CAD build for the part. Positions are in the model's coordinates, mm. Round coordinates to 2 decimals unless told otherwise and drop trailing zeros. Loops run counter-clockwise (first coordinate to the right, second up) from the corner with the lowest first, then second, coordinate; pieces in that order, holes last.
from build123d import *

# Parameters (mm, degrees)
SKETCH_W      = 56
SKETCH_H      = 306
PAD_DEPTH     = 3
SKETCH001_W   = 8
SKETCH001_H   = 3
SKETCH001_W_2 = 3
SKETCH001_H_2 = 20
POCKET_DEPTH  = 3.001


with BuildPart() as part:
    # Sketch → Pad (new body)
    with BuildSketch(Plane.XY):
        with Locations((28, 153)):
            Rectangle(SKETCH_W, SKETCH_H)
    extrude(amount=PAD_DEPTH)

    # Sketch001 (on Face6 of Pad) → Pocket (cut, through all)
    with BuildSketch(Plane.XY.offset(3)):
        with Locations((4, 1.5)):
            Rectangle(SKETCH001_W, SKETCH001_H)
        with Locations((20, 1.5)):
            Rectangle(SKETCH001_W, SKETCH001_H)
        with Locations((36, 1.5)):
            Rectangle(SKETCH001_W, SKETCH001_H)
        with Locations((52, 1.5)):
            Rectangle(SKETCH001_W, SKETCH001_H)
        with Locations((4, 304.5)):
            Rectangle(SKETCH001_W, SKETCH001_H)
        with Locations((20, 304.5)):
            Rectangle(SKETCH001_W, SKETCH001_H)
        with Locations((36, 304.5)):
            Rectangle(SKETCH001_W, SKETCH001_H)
        with Locations((52, 304.5)):
            Rectangle(SKETCH001_W, SKETCH001_H)
        with Locations((1.5, 33)):
            Rectangle(SKETCH001_W_2, SKETCH001_H_2)
        with Locations((1.5, 73)):
            Rectangle(SKETCH001_W_2, SKETCH001_H_2)
        with Locations((1.5, 113)):
            Rectangle(SKETCH001_W_2, SKETCH001_H_2)
        with Locations((1.5, 153)):
            Rectangle(SKETCH001_W_2, SKETCH001_H_2)
        with Locations((1.5, 193)):
            Rectangle(SKETCH001_W_2, SKETCH001_H_2)
        with Locations((1.5, 233)):
            Rectangle(SKETCH001_W_2, SKETCH001_H_2)
        with Locations((1.5, 273)):
            Rectangle(SKETCH001_W_2, SKETCH001_H_2)
        with Locations((54.5, 33)):
            Rectangle(SKETCH001_W_2, SKETCH001_H_2)
        with Locations((54.5, 73)):
            Rectangle(SKETCH001_W_2, SKETCH001_H_2)
        with Locations((54.5, 113)):
            Rectangle(SKETCH001_W_2, SKETCH001_H_2)
        with Locations((54.5, 153)):
            Rectangle(SKETCH001_W_2, SKETCH001_H_2)
        with Locations((54.5, 193)):
            Rectangle(SKETCH001_W_2, SKETCH001_H_2)
        with Locations((54.5, 233)):
            Rectangle(SKETCH001_W_2, SKETCH001_H_2)
        with Locations((54.5, 273)):
            Rectangle(SKETCH001_W_2, SKETCH001_H_2)
    extrude(amount=-POCKET_DEPTH, mode=Mode.SUBTRACT)


solid = part.part
Item 1: Wall check: L1, parallel to X at y = 233.5, z = 2.5; L2, parallel to Y at x = 49.5, z = 0.7. Give the ranges that are in metal, low to high.
Verdict:
L1: x = 3 to 53
L2: y = 3 to 303
Item 2: Cut at A-A (y = 112.5). List the corners of the cut face in (x, z).
Verdict:
outline: (3, 0) - (53, 0) - (53, 3) - (3, 3) - close
Item 3: Flat gauge pins, fed straight in: P1, Ø0.9, axis at x = 2, z = 2, coming from the -Y side; P2, Ø1.5, axis at y = 156.5, z = 2, coming from the -X side; P3, Ø1.5, axis at x = 54.5, z = 2, coming from the +Y side. Where does each tip first touch, or does it go through?
Verdict:
P1: stops at y = 3
P2: stops at x = 3
P3: stops at y = 303
